Source: CAD feature listing. Evaluate the final solid. Frame: model axes, mm. A direction names the side the tool comes from. Coordinates: 2 decimals unless noted, no trailing zeros. Order: outer loops, then holes, each group sorted by start corner. A loop starts at its lowest first (then second) coordinate and runs counter-clockwise, first axis right, second up.
```python
from build123d import *

# Parameters (mm, degrees)
SKETCH1_R           = 15
BOSS_EXTRUDE6_DEPTH = 15
BOSS_EXTRUDE7_DEPTH = 15
SKETCH5_R           = 7.5
BOSS_EXTRUDE8_DEPTH = 30
SKETCH6_R           = 50
BOSS_EXTRUDE9_DEPTH = 15
CUT_EXTRUDE1_DEPTH  = 15
SKETCH8_R           = 15
CUT_EXTRUDE2_DEPTH  = 16
SKETCH9_W           = 8
SKETCH9_H           = 6
CUT_EXTRUDE3_DEPTH  = 46


with BuildPart() as part:
    # Sketch1 → Boss-Extrude6 (new body, symmetric)
    with BuildSketch(Plane(origin=(0, 0, 0), x_dir=(1, 0, 0), z_dir=(0, 1, 0))):
        with BuildLine():
            ThreePointArc((40.625, 29.148059541), (-50, 0), (40.625, -29.148059541))
            ThreePointArc((40.625, -29.148059541), (25, 0), (40.625, 29.148059541))
        make_face()
        Circle(SKETCH1_R, mode=Mode.SUBTRACT)
    extrude(amount=BOSS_EXTRUDE6_DEPTH, both=True)

    # Sketch4 → Boss-Extrude7 (add)
    with BuildSketch(Plane(origin=(0, 0, 0), x_dir=(1, 0, 0), z_dir=(0, 1, 0))):
        with BuildLine():
            Line((65, 7.5), (25.813014172, 7.5))
            ThreePointArc((25.813014172, 7.5), (25, 0), (25.813014172, -7.5))
            Line((25.813014172, -7.5), (65, -7.5))
            ThreePointArc((65, -7.5), (72.5, 0), (65, 7.5))
        make_face()
    extrude(amount=-BOSS_EXTRUDE7_DEPTH)

    # Sketch5 → Boss-Extrude8 (add)
    with BuildSketch(Plane(origin=(0, 15, 0), x_dir=(1, 0, 0), z_dir=(0, 1, 0))):
        with Locations((65, 0)):
            Circle(SKETCH5_R)
    extrude(amount=-BOSS_EXTRUDE8_DEPTH)

    # Sketch6 → Boss-Extrude9 (add)
    with BuildSketch(Plane.XZ.offset(15)):
        Circle(SKETCH6_R)
    extrude(amount=BOSS_EXTRUDE9_DEPTH)

    # Sketch7 → Cut-Extrude1 (cut)
    with BuildSketch(Plane(origin=(0, 15, 0), x_dir=(1, 0, 0), z_dir=(0, 1, 0))):
        with BuildLine():
            Line((0, 0), (25, -43.301270189))
            ThreePointArc((25, -43.301270189), (33.566925673, -37.057543103), (40.625, -29.148059541))
            ThreePointArc((40.625, -29.148059541), (25, 0), (40.625, 29.148059541))
            ThreePointArc((40.625, 29.148059541), (33.566925673, 37.057543103), (25, 43.301270189))
            Line((25, 43.301270189), (0, 0))
        make_face()
    extrude(amount=-CUT_EXTRUDE1_DEPTH, mode=Mode.SUBTRACT)

    # Sketch8 → Cut-Extrude2 (cut, through all)
    with BuildSketch(Plane(origin=(0, -15, 0), x_dir=(1, 0, 0), z_dir=(0, 1, 0))):
        Circle(SKETCH8_R)
    extrude(amount=-CUT_EXTRUDE2_DEPTH, mode=Mode.SUBTRACT)

    # Sketch9 → Cut-Extrude3 (cut, through all)
    with BuildSketch(Plane(origin=(0, 15, 0), x_dir=(1, 0, 0), z_dir=(0, 1, 0))):
        with Locations((-15, 0)):
            Rectangle(SKETCH9_W, SKETCH9_H)
    extrude(amount=-CUT_EXTRUDE3_DEPTH, mode=Mode.SUBTRACT)


solid = part.part
```
1. Pin query (flat end, axial travel): P1, Ø3, axis at x = -27, y = 10.5, coming from the -Z side; P2, Ø3.5, axis at x = -16, y = -2.5, coming from the +Z side; P3, Ø17.5, axis at x = 39, z = -19, coming from the +Y side; P4, Ø5, axis at y = -2, z = -0.5, coming from the +X side. Return the tip coordinate at first contact, or that it passes through.
Findings:
P1: stops at z = -43.01
P2: stops at z = 47.93
P3: stops at y = 0
P4: stops at x = 72.5
2. Section query D-D on z = 19. Return loops of the section in (x, y).
Findings:
outline: (-46.25, -30) - (46.25, -30) - (46.25, -15) - (30.61, -15) - (30.61, 0) - (10.97, 0) - (10.97, 15) - (-46.25, 15) - close
3. Section query C-C on x = 59. Return loops of the section in (y, z).
Findings:
outline: (-15, -7.5) - (0, -7.5) - (0, -4.5) - (15, -4.5) - (15, 4.5) - (0, 4.5) - (0, 7.5) - (-15, 7.5) - close
4. Ray query, line 1 (Y direction, x = 38, z = 17.5); line 2 (Z direction, x = -3.5, y = -12); line 3 (X direction, y = -24, z = 11.5). Return the intervals inside material, ascending.
Findings:
line 1: y = -30 to -15
line 2: z = -49.88 to -14.59, 14.59 to 49.88
line 3: x = -48.66 to -9.63, 9.63 to 48.66
5. Section query B-B on y = -6. Return loops of the section in (x, z) (3 decimals), plus the area to 3 significant figures.
Findings:
outline: (25.813, -7.5) - (65, -7.5) arc R7.5 ccw to (65, 7.5) - (25.813, 7.5) arc R35 cw to (40.625, 29.148) arc R50 ccw (long way) to (40.625, -29.148) arc R35 cw to start; hole (-19, -3) - (-14.697, -3) arc R15 ccw (long way) to (-14.697, 3) - (-19, 3) - close
area: 6,790 mm2
6. Access query for faces 4 (the face through (-17, -7, 3)), 5 (the face through (65, 15, 0)), 6 (the face through (46, -7, -7.5)). Directions: +Z, -Z, +X, -X, +Y, -Y. A direction counts if a zero-diameter tool reaches every point of the face in a straight line with its end or side. Return the directions, or none.
Findings:
face 4: +Y, -Y
face 5: +Z, -Z, +X, -X, +Y
face 6: +X, +Y
7. Draft query along X for faces 1 (the face through (37, -15, -16)), 2 (the face through (16.373, 7.605, -28.358)), 3 (the face through (-17, -7, -3)). Return one class per face: released by +X, released by -X, zero draft, split by the parting line, or undercut.
Findings:
face 1: zero draft
face 2: released by +X
face 3: undercut
8. Section query A-A on x = 0. Return loops of the section in (y, z), plus the area to 3 significant figures.
Findings:
outline: (-30, -50) - (15, -50) - (15, -15) - (-30, -15) - close; (-30, 15) - (15, 15) - (15, 50) - (-30, 50) - close
area: 3,150 mm2
